```python
from build123d import *

# Parameters (mm, degrees)
BOSS_EXTRUDE1_DEPTH = 90
CUT_EXTRUDE1_REACH  = 172.789
SKETCH2_R           = 11


with BuildPart() as part:
    # Sketch1 → Boss-Extrude1 (new, symmetric)
    with BuildSketch(Plane.XY):
        with BuildLine():
            Line((-45, 75), (-45, -75))
            Line((-45, -75), (45, -75))
            Line((45, -75), (45, -69))
            ThreePointArc((45, -69), (43.242640687, -64.757359313), (39, -63))
            Line((39, -63), (-21, -63))
            ThreePointArc((-21, -63), (-29.485281374, -59.485281374), (-33, -51))
            Line((-33, -51), (-33, 69))
            ThreePointArc((-33, 69), (-34.757359313, 73.242640687), (-39, 75))
            Line((-39, 75), (-45, 75))
        make_face()
    extrude(amount=BOSS_EXTRUDE1_DEPTH, both=True)

    # Sketch2 → Cut-Extrude1 (cut, up to next)
    with BuildSketch(Plane(origin=(0, -63, 0), x_dir=(1, 0, 0), z_dir=(0, 1, 0)), mode=Mode.PRIVATE) as cut_extrude1_sk1:
        with Locations(Location((5, -60, 0), (0, 0, 180))):
            Circle(SKETCH2_R)
    cut_extrude1_tool1 = extrude(cut_extrude1_sk1.sketch, amount=-CUT_EXTRUDE1_REACH, mode=Mode.PRIVATE) & part.part
    # Sketch2 → Cut-Extrude1 (cut, up to next)
    with BuildSketch(Plane(origin=(0, -63, 0), x_dir=(1, 0, 0), z_dir=(0, 1, 0)), mode=Mode.PRIVATE) as cut_extrude1_sk2:
        with Locations(Location((5, 60, 0), (0, 0, 180))):
            Circle(SKETCH2_R)
    cut_extrude1_tool2 = extrude(cut_extrude1_sk2.sketch, amount=-CUT_EXTRUDE1_REACH, mode=Mode.PRIVATE) & part.part
    add(cut_extrude1_tool1.solids().sort_by_distance((5, -63, 60))[0], mode=Mode.SUBTRACT)
    add(cut_extrude1_tool2.solids().sort_by_distance((5, -63, -60))[0], mode=Mode.SUBTRACT)


solid = part.part
```
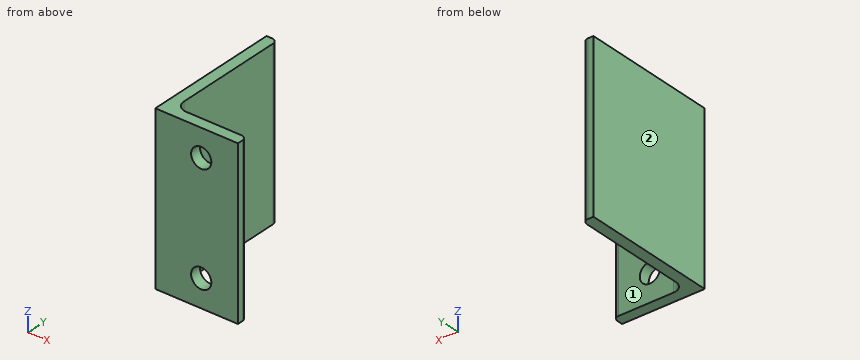
The listing builds one solid part. Answer for the finished solid, in the listing's coordinates (mm). Face numbers are marked on the shaded views. A direction names the side the tool comes from. Give positions to 0.01 mm unless a question says otherwise; leave off trailing zeros. Order: outer loops, then holes, each group sorted by start corner. A loop starts at its lowest first (then second) coordinate and runs counter-clockwise, first axis right, second up. Notation, with made-up numbers: M -1,88.25 L 24,88.25 A20 ccw 24,110.25 Z; hole C 25.5,28 d7. An arc over 180 degrees is marked long. Put each result on its own line as item: value. Start each with the question number.
Item 1: The part is cut by section D-D, the plane y = 2.5. Determine the outline of the cut face in (x, z).
Item 2: Find the intervals of material crossed by line 1 along Z through (x, y) = (5, -71.5); line 2 along Y through (x, z) = (34, -24.5); line 3 along X through (y, z) = (-49, -24), in increasing order.
Item 3: The part is cut by section B-B, the plane z = -60. Determine the outline of the cut face in (x, y).
Item 4: The part is cut by section C-C, the plane z = 41. Determine the outline of the cut face in (x, y).
Item 5: Which of the six approach directions +Z, -Z, +X, -X, +Y, -Y give full straight-line access (tool end or side, diameter ignored) to the marked faces 1 and 2?
Item 6: The part is cut by section A-A, the plane x = 5. Determine the outline of the cut face in (y, z), and give its area (3 significant figures).
Item 7: Flat-ended cylindrical pins translate along their axes: P1, Ø3, axis at x = -34.5, z = -68.5, coming from the +Y side; P2, Ø18, axis at x = 20.5, z = -13, coming from the +Y side; P3, Ø12, axis at x = -34.5, z = -22, coming from the +Y side. Find the tip coordinate at first contact, or state that the pin passes through.
Answer key:
1. outline: M -45,-90 L -33,-90 L -33,90 L -45,90 Z
2. line 1: z = -90 to -71, -49 to 49, 71 to 90
2. line 2: y = -75 to -63
2. line 3: x = -45 to -33
3. outline: M -45,-75 L -6,-75 L -6,-63 L -21,-63 A12 cw -33,-51 L -33,69 A6 ccw -39,75 L -45,75 Z; M 16,-75 L 45,-75 L 45,-69 A6 ccw 39,-63 L 16,-63 Z
4. outline: M -45,-75 L 45,-75 L 45,-69 A6 ccw 39,-63 L -21,-63 A12 cw -33,-51 L -33,69 A6 ccw -39,75 L -45,75 Z
5. face 1: +Z, -Z, +X, +Y
5. face 2: +Z, -Z, -X, +Y, -Y
6. outline: M -75,-90 L -63,-90 L -63,-71 L -75,-71 Z; M -75,-49 L -63,-49 L -63,49 L -75,49 Z; M -75,71 L -63,71 L -63,90 L -75,90 Z
6. area: 1,630 mm²
7. P1: stops at y = 74.2
7. P2: stops at y = -63
7. P3: stops at y = 75
